from build123d import *

# Parameters (mm, degrees)
EXTRUDE_1_DEPTH     = 2.9
CUT_EXTRUDE_1_REACH = 43.764
SKETCH_2_R          = 1
EXTRUDE_START       = 1.2
SKETCH_3_W          = 29.092354585
SKETCH_3_H          = 29.600355601
EXTRUDE_2_DEPTH     = 1.2
CUT_EXTRUDE_2_REACH = 43.864
SKETCH_4_W          = 27.4
SKETCH_4_H          = 19.4
SKETCH_5_W          = 14
SKETCH_5_H          = 5.100177801
SKETCH_5_H_2        = 5.1001778
CUT_EXTRUDE_3_DEPTH = 1.8
SKETCH_6_W          = 4.41346869
SKETCH_6_H          = 1
EXTRUDE_3_DEPTH     = 5.8
SKETCH_8_W          = 27.4
SKETCH_8_H          = 1.1
EXTRUDE_4_DEPTH     = 4.5
SKETCH_9_R          = 2
CUT_EXTRUDE_4_DEPTH = 1.5
SKETCH_10_W         = 0.8
SKETCH_10_H         = 14.9
EXTRUDE_5_DEPTH     = 1.8


with BuildPart() as part:
    # 草图1 → 凸台-拉伸1 (new body)
    with BuildSketch(Plane.XY.offset(12.2)):
        with BuildLine():
            Line((28.20505461, 1.887299975), (-0.887299975, 1.887299975))
            ThreePointArc((-0.887299975, 1.887299975), (-1.594406756, 1.594406756), (-1.887299975, 0.887299975))
            Line((-1.887299975, 0.887299975), (-1.887299975, -28.713055626))
            ThreePointArc((-1.887299975, -28.713055626), (-1.594406756, -29.420162407), (-0.887299975, -29.713055626))
            Line((-0.887299975, -29.713055626), (12.510283784, -29.713055626))
            Line((12.510283784, -29.713055626), (16.923752474, -29.713055626))
            Line((16.923752474, -29.713055626), (28.20505461, -29.713055626))
            ThreePointArc((28.20505461, -29.713055626), (28.912161391, -29.420162407), (29.20505461, -28.713055626))
            Line((29.20505461, -28.713055626), (29.20505461, 0.887299975))
            ThreePointArc((29.20505461, 0.887299975), (28.912161391, 1.594406756), (28.20505461, 1.887299975))
        make_face()
    extrude(amount=EXTRUDE_1_DEPTH)

    # 草图2 → 切除-拉伸1 (cut, up to next)
    with BuildSketch(Plane(origin=(0, 0, 12.2), x_dir=(-1, 0, 0), z_dir=(0, 0, -1)), mode=Mode.PRIVATE) as cut_extrude_1_sk1:
        with Locations((-25.308877318, -2.012877826)):
            Circle(SKETCH_2_R)
    cut_extrude_1_tool1 = extrude(cut_extrude_1_sk1.sketch, amount=-CUT_EXTRUDE_1_REACH, mode=Mode.PRIVATE) & part.part
    # 草图2 → 切除-拉伸1 (cut, up to next)
    with BuildSketch(Plane(origin=(0, 0, 12.2), x_dir=(-1, 0, 0), z_dir=(0, 0, -1)), mode=Mode.PRIVATE) as cut_extrude_1_sk2:
        with Locations((-25.308877318, -25.812877826)):
            Circle(SKETCH_2_R)
    cut_extrude_1_tool2 = extrude(cut_extrude_1_sk2.sketch, amount=-CUT_EXTRUDE_1_REACH, mode=Mode.PRIVATE) & part.part
    # 草图2 → 切除-拉伸1 (cut, up to next)
    with BuildSketch(Plane(origin=(0, 0, 12.2), x_dir=(-1, 0, 0), z_dir=(0, 0, -1)), mode=Mode.PRIVATE) as cut_extrude_1_sk3:
        with Locations((-2.008877318, -25.812877826)):
            Circle(SKETCH_2_R)
    cut_extrude_1_tool3 = extrude(cut_extrude_1_sk3.sketch, amount=-CUT_EXTRUDE_1_REACH, mode=Mode.PRIVATE) & part.part
    # 草图2 → 切除-拉伸1 (cut, up to next)
    with BuildSketch(Plane(origin=(0, 0, 12.2), x_dir=(-1, 0, 0), z_dir=(0, 0, -1)), mode=Mode.PRIVATE) as cut_extrude_1_sk4:
        with Locations(Location((-2.008877318, -2.012877826, 0), (0, 0, 180))):
            Circle(SKETCH_2_R)
    cut_extrude_1_tool4 = extrude(cut_extrude_1_sk4.sketch, amount=-CUT_EXTRUDE_1_REACH, mode=Mode.PRIVATE) & part.part
    add(cut_extrude_1_tool1.solids().sort_by_distance((25.308877, -2.012878, 12.2))[0], mode=Mode.SUBTRACT)
    add(cut_extrude_1_tool2.solids().sort_by_distance((25.308877, -25.812878, 12.2))[0], mode=Mode.SUBTRACT)
    add(cut_extrude_1_tool3.solids().sort_by_distance((2.008877, -25.812878, 12.2))[0], mode=Mode.SUBTRACT)
    add(cut_extrude_1_tool4.solids().sort_by_distance((2.008877, -2.012878, 12.2))[0], mode=Mode.SUBTRACT)

    # 草图3 → 凸台-拉伸2 (add)
    with BuildSketch(Plane(origin=(0, 0, 12.2), x_dir=(-1, 0, 0), z_dir=(0, 0, -1)).offset(EXTRUDE_START)):
        with BuildLine():
            Line((0.887299975, 1.887299975), (-28.20505461, 1.887299975))
            ThreePointArc((-28.20505461, 1.887299975), (-28.912161391, 1.594406756), (-29.20505461, 0.887299975))
            Line((-29.20505461, 0.887299975), (-29.20505461, -28.713055626))
            ThreePointArc((-29.20505461, -28.713055626), (-28.912161391, -29.420162407), (-28.20505461, -29.713055626))
            Line((-28.20505461, -29.713055626), (0.887299975, -29.713055626))
            ThreePointArc((0.887299975, -29.713055626), (1.594406756, -29.420162407), (1.887299975, -28.713055626))
            Line((1.887299975, -28.713055626), (1.887299975, 0.887299975))
            ThreePointArc((1.887299975, 0.887299975), (1.594406756, 1.594406756), (0.887299975, 1.887299975))
        make_face()
        with Locations((-13.658877318, -13.912877826)):
            Rectangle(SKETCH_3_W, SKETCH_3_H, mode=Mode.SUBTRACT)
    extrude(amount=-EXTRUDE_2_DEPTH)

    # 草图4 → 切除-拉伸2 (cut, up to next)
    with BuildSketch(Plane.XY.offset(15.1), mode=Mode.PRIVATE) as cut_extrude_2_sk1:
        with Locations((13.658877318, -13.912877826)):
            Rectangle(SKETCH_4_W, SKETCH_4_H)
    cut_extrude_2_tool1 = extrude(cut_extrude_2_sk1.sketch, amount=-CUT_EXTRUDE_2_REACH, mode=Mode.PRIVATE) & part.part
    add(cut_extrude_2_tool1.solids().sort_by_distance((13.658877, -13.912878, 15.1))[0], mode=Mode.SUBTRACT)

    # 草图5 → 切除-拉伸3 (cut)
    with BuildSketch(Plane(origin=(0, 0, 12.2), x_dir=(-1, 0, 0), z_dir=(0, 0, -1))):
        with Locations((-13.658877318, -1.662788926)):
            Rectangle(SKETCH_5_W, SKETCH_5_H)
        with Locations((-13.658877318, -26.162966726)):
            Rectangle(SKETCH_5_W, SKETCH_5_H_2)
    extrude(amount=-CUT_EXTRUDE_3_DEPTH, mode=Mode.SUBTRACT)

    # 草图6 → 凸台-拉伸3 (add)
    with BuildSketch(Plane(origin=(0, 0, 11), x_dir=(-1, 0, 0), z_dir=(0, 0, -1))):
        with Locations((-14.717018129, -29.213055626)):
            Rectangle(SKETCH_6_W, SKETCH_6_H)
    extrude(amount=EXTRUDE_3_DEPTH)

    # 草图8 → 凸台-拉伸4 (add)
    with BuildSketch(Plane(origin=(0, -4.212877826, 0), x_dir=(1, 0, 0), z_dir=(0, 1, 0))):
        with Locations((13.658877318, -14.55)):
            Rectangle(SKETCH_8_W, SKETCH_8_H)
    extrude(amount=-EXTRUDE_4_DEPTH)

    # 草图9 → 切除-拉伸4 (cut)
    with BuildSketch(Plane.XY.offset(15.1)):
        with Locations((25.308877318, -2.012877826)):
            Circle(SKETCH_9_R)
        with Locations((2.008877318, -2.012877826)):
            Circle(SKETCH_9_R)
        with Locations((2.008877318, -25.812877826)):
            Circle(SKETCH_9_R)
        with Locations((25.308877318, -25.812877826)):
            Circle(SKETCH_9_R)
    extrude(amount=-CUT_EXTRUDE_4_DEPTH, mode=Mode.SUBTRACT)

    # 草图10 → 凸台-拉伸5 (add)
    with BuildSketch(Plane(origin=(-0.041122682, 0, 0), x_dir=(0, 0, -1), z_dir=(1, 0, 0))):
        with Locations((-14.7, -16.162877826)):
            Rectangle(SKETCH_10_W, SKETCH_10_H)
    extrude_5 = extrude(amount=EXTRUDE_5_DEPTH)

    # 镜向1: 凸台-拉伸5 across plane
    add(extrude_5.mirror(Plane(origin=(13.658877318, 0, 0), x_dir=(0, 0, 1), z_dir=(1, 0, 0))))


solid = part.part
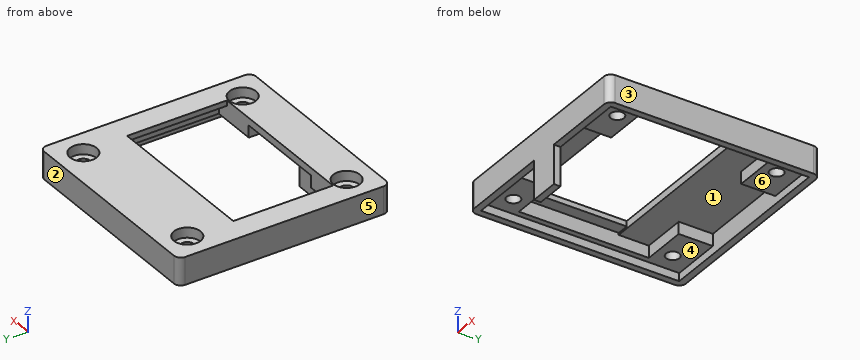
Read the model definition and answer for the solid it produces. Units are mm, in the model's axes. Face numbers are marked on the shaded views. A direction names the side the tool comes from. Give positions to 0.01 mm unless a question says otherwise; leave off trailing zeros. Write each loop counter-clockwise with the first axis right and the second up, starting at its lowest first coordinate (ties: lowest second). Pieces come first, ordered by that corner, then holes. Notation, with made-up numbers: (7.25, 24) - (53.25, 24) arc R16 ccw to (53.25, 43) - close; hole circle Ø7 at (10.5, 53.5). An arc over 180 degrees is marked (long way). Return JSON: item names as keys, results as strings.
Q1. Given P1, Ø6, axis at x = 2.5, y = -21.5, coming from the -Z side; P2, Ø8, axis at x = 22.5, y = -2.5, coming from the -Z side; P3, Ø0.5, axis at y = -29.5, z = 7, coming from the +X side; P4, Ø1.2, axis at x = 25.5, y = -26, coming from the +Z side, each flat-ended and moving along its own axis, determine where each tip first touches the part or whether it passes through.
Reply:
{"P1": "z = 12.2", "P2": "z = 11", "P3": "x = 16.92", "P4": "through"}
Q2. A cutting plane is placed at B-B, the plane y = -12. Determine the outline of the cut face in (x, z).
Reply:
{"outline": "(-1.89, 11) - (-0.89, 11) - (-0.89, 12.2) - (-0.04, 12.2) - (-0.04, 14.3) - (1.76, 14.3) - (1.76, 15.1) - (-1.89, 15.1) - close; (25.56, 14.3) - (27.36, 14.3) - (27.36, 12.2) - (28.21, 12.2) - (28.21, 11) - (29.21, 11) - (29.21, 15.1) - (25.56, 15.1) - close"}
Q3. A cutting plane is placed at D-D, the plane y = -6. Determine the outline of the cut face in (x, z).
Reply:
{"outline": "(-1.89, 11) - (-0.89, 11) - (-0.89, 12.2) - (-0.04, 12.2) - (-0.04, 14) - (27.36, 14) - (27.36, 12.2) - (28.21, 12.2) - (28.21, 11) - (29.21, 11) - (29.21, 15.1) - (-1.89, 15.1) - close"}
Q4. Consider line 1 along X through (y, z) = (-22.5, 12.5); line 2 along Y through (x, z) = (0.5, 12); line 3 along Y through (x, z) = (13, 14.5). Determine where each line is inside the solid, lowest interval first. Write a range as [from, to].
Reply:
{"line 1": "[-1.89, -0.04], [27.36, 29.21]", "line 2": "[-29.71, -28.71], [0.89, 1.89]", "line 3": "[-29.71, -23.61], [-8.71, 1.89]"}
Q5. A cutting plane is placed at C-C, the plane z = 11.75. Determine the outline of the cut face in (x, y).
Reply:
{"outline": "(-1.89, -28.71) arc R1 ccw to (-0.89, -29.71) - (28.21, -29.71) arc R1 ccw to (29.21, -28.71) - (29.21, 0.89) arc R1 ccw to (28.21, 1.89) - (-0.89, 1.89) arc R1 ccw to (-1.89, 0.89) - close; hole (-0.89, -28.71) - (28.21, -28.71) - (28.21, 0.89) - (-0.89, 0.89) - close"}
Q6. For the marked faces 5 and 6, determine the directions among +Z, -Z, +X, -X, +Y, -Y from which every point of the face is accessible in a straight line to the end or side of a thin tool.
Reply:
{"face 5": "+Z, -Z, -X, +Y, -Y", "face 6": "-Z"}
Q7. For a pull along Y with two mould halves and no side action, classify the marked faces 1, 2, 3 and 4 as released by +Y, released by -Y, zero draft, split by the parting line, or undercut.
Reply:
{"face 1": "undercut", "face 2": "released by +Y", "face 3": "zero draft", "face 4": "undercut"}
Q8. A cutting plane is placed at A-A, the plane x = 11. Determine the outline of the cut face in (y, z), and give its area (3 significant figures).
Reply:
{"outline": "(-29.71, 11) - (-28.71, 11) - (-28.71, 14) - (-23.61, 14) - (-23.61, 15.1) - (-29.71, 15.1) - close; (-8.71, 14) - (0.89, 14) - (0.89, 11) - (1.89, 11) - (1.89, 15.1) - (-8.71, 15.1) - close", "area": "24.4 mm²"}
